```python
from build123d import *

# Parameters (mm, degrees)
ESQUISSE1_R             = 2
BOSS_EXTRU_1_DEPTH      = 10
ESQUISSE3_W             = 60
ESQUISSE3_H             = 3.628659563
BOSS_EXTRU_2_DEPTH      = 10
ENL_V_MAT_EXTRU_1_REACH = 23.129
ESQUISSE4_R             = 2


with BuildPart() as part:
    # Esquisse1 → Boss.-Extru.1 (new body)
    with BuildSketch(Plane.XY):
        with BuildLine():
            Line((-21, 3.5), (-21, -3.5))
            Line((-21, -3.5), (-13.555441712, -3.5))
            Line((-13.555441712, -3.5), (-13.555441712, 3.5))
            ThreePointArc((-13.555441712, 3.5), (0, 14), (13.555441712, 3.5))
            Line((13.555441712, 3.5), (13.555441712, -3.5))
            Line((13.555441712, -3.5), (21, -3.5))
            Line((21, -3.5), (21, 3.5))
            Line((21, 3.5), (17.277720856, 3.5))
            ThreePointArc((17.277720856, 3.5), (0, 17.628659563), (-17.277720856, 3.5))
            Line((-17.277720856, 3.5), (-21, 3.5))
        make_face()
        with Locations((-17.5, 0)):
            Circle(ESQUISSE1_R, mode=Mode.SUBTRACT)
        with Locations((17.5, 0)):
            Circle(ESQUISSE1_R, mode=Mode.SUBTRACT)
    extrude(amount=BOSS_EXTRU_1_DEPTH)

    # Esquisse3 → Boss.-Extru.2 (add)
    with BuildSketch(Plane.XY):
        with Locations((0, 15.814329781)):
            Rectangle(ESQUISSE3_W, ESQUISSE3_H)
    extrude(amount=BOSS_EXTRU_2_DEPTH)

    # Esquisse4 → Enlèv. mat.-Extru.1 (cut, up to next)
    with BuildSketch(Plane(origin=(0, 17.628659563, 0), x_dir=(1, 0, 0), z_dir=(0, 1, 0)), mode=Mode.PRIVATE) as enl_v_mat_extru_1_sk1:
        with Locations((-25, -5)):
            Circle(ESQUISSE4_R)
    enl_v_mat_extru_1_tool1 = extrude(enl_v_mat_extru_1_sk1.sketch, amount=-ENL_V_MAT_EXTRU_1_REACH, mode=Mode.PRIVATE) & part.part
    add(enl_v_mat_extru_1_tool1.solids().sort_by_distance((-25, 17.62866, 5))[0], mode=Mode.SUBTRACT)
    # Esquisse4 → Enlèv. mat.-Extru.1 (cut, up to next)
    with BuildSketch(Plane(origin=(0, 17.628659563, 0), x_dir=(1, 0, 0), z_dir=(0, 1, 0)), mode=Mode.PRIVATE) as enl_v_mat_extru_1_sk2:
        with Locations((25, -5)):
            Circle(ESQUISSE4_R)
    enl_v_mat_extru_1_tool2 = extrude(enl_v_mat_extru_1_sk2.sketch, amount=-ENL_V_MAT_EXTRU_1_REACH, mode=Mode.PRIVATE) & part.part
    add(enl_v_mat_extru_1_tool2.solids().sort_by_distance((25, 17.62866, 5))[0], mode=Mode.SUBTRACT)


solid = part.part
```
Geometry: final body of the model. Coordinates: model frame, mm. A direction names the side the tool comes from. Coordinates: 2 decimals unless noted, no trailing zeros. Order: outer loops, then holes, each group sorted by start corner. A loop starts at its lowest first (then second) coordinate and runs counter-clockwise, first axis right, second up. Notation, with made-up numbers: M 58,10.5 L 92,10.5 A32 cw 92,37.5 Z; hole C -16.5,78 d6. An arc over 180 degrees is marked long. Answer in a Markdown table with one row per item. Add a question column.
Q1. Mould query, pull axis X, two halves, no side actions, for faces 5 (the flat face through (19, 3.5, 5)), 6 (the flat face through (13.555, 0, 5)), 7 (the flat face through (-21, 0, 5)). Classes: released by +X, released by -X, zero draft, split by the parting line, or undercut.
Q2. Contact query for flat-ended pins moving along their axis: P1, Ø3, axis at y = 0.5, z = 4.5, coming from the +X side; P2, Ø1.5, axis at x = 6.5, z = 6, coming from the -Y side; P3, Ø2, axis at y = 0, z = 5, coming from the -X side. Output: stop coordinate, or through.
Q3. Section query D-D on y = 15.5. Return the cut outline in (x, z).
Q4. Section query B-B on x = -25. Return the cut outline in (y, z).
Q5. Section query A-A on z = 5. Return the cut outline in (x, y), and give its area (3 significant figures).
Q6. Reachability of faces 1 (the flat face through (20, 14, 5)), 2 (the flat face through (21, 0, 5)), 3 (the flat face through (-19, 3.5, 5)), 4 (the cylindrical face through (23.4, 15.8, 6.2)) from +Z, -Z, +X, -X, +Y, -Y: full face, straight path, thin tool, end or side. Return the list, or none.
Q7. Section query C-C on z = 2. Return the cut outline in (x, y).
Q8. Line query: L1, parallel to X at y = 15.6, z = 5; L2, parallel to Z at x = 25, y = 16.95; L3, parallel to X at y = 3, z = 2. Output: solid intervals per line, ascending.
Completed:
| question | item | result |
|---|---|---|
| 1 | face 5 | zero draft |
| 1 | face 6 | undercut |
| 1 | face 7 | released by -X |
| 2 | P1 | stops at x = 21 |
| 2 | P2 | stops at y = 11.98 |
| 2 | P3 | stops at x = -21 |
| 3 | outline | M -30,0 L 30,0 L 30,10 L -30,10 Z; hole C -25,5 d4; hole C 25,5 d4 |
| 4 | outline | M 14,0 L 17.63,0 L 17.63,3 L 14,3 Z; M 14,7 L 17.63,7 L 17.63,10 L 14,10 Z |
| 5 | outline | M -30,14 L -27,14 L -27,17.63 L -30,17.63 Z; M -23,14 L -10.71,14 A17.63 ccw -17.28,3.5 L -21,3.5 L -21,-3.5 L -13.56,-3.5 L -13.56,3.5 A14 cw 13.56,3.5 L 13.56,-3.5 L 21,-3.5 L 21,3.5 L 17.28,3.5 A17.63 ccw 10.71,14 L 23,14 L 23,17.63 L -23,17.63 Z; M 27,14 L 30,14 L 30,17.63 L 27,17.63 Z; hole C -17.5,0 d4; hole C 17.5,0 d4 |
| 5 | area | 369 mm2 |
| 6 | face 1 | +Z, -Z, +X |
| 6 | face 2 | +Z, -Z, +X, -Y |
| 6 | face 3 | +Z, -Z, -X |
| 6 | face 4 | +Y, -Y |
| 7 | outline | M -30,14 L -10.71,14 A17.63 ccw -17.28,3.5 L -21,3.5 L -21,-3.5 L -13.56,-3.5 L -13.56,3.5 A14 cw 13.56,3.5 L 13.56,-3.5 L 21,-3.5 L 21,3.5 L 17.28,3.5 A17.63 ccw 10.71,14 L 30,14 L 30,17.63 L -30,17.63 Z; hole C -17.5,0 d4; hole C 17.5,0 d4 |
| 8 | L1 | x = -30 to -27, -23 to 23, 27 to 30 |
| 8 | L2 | z = 0 to 3, 7 to 10 |
| 8 | L3 | x = -21 to -13.56, 13.56 to 21 |
